Work out the finished part from the listing and answer in its coordinate system (mm). Face numbers are marked on the shaded views. A direction names the side the tool comes from. Coordinates: 2 decimals unless noted, no trailing zeros. Order: outer loops, then holes, each group sorted by start corner. A loop starts at its lowest first (then second) coordinate and runs counter-clockwise, first axis right, second up.
1. Determine the mould class of the marked faces 1, 2, 3 and 4 for opening direction X: +X half, -X half, draft (parallel to the pull), parting line (faces both ways), or undercut.
2. The part is cut by section B-B, the plane x = -6. Give the vertices of the cut face in (y, z), then the cut area to 3 significant figures.
3. Find the intervals of material crossed by probe 1 along X at (y, z) = (6, 0.45); probe 2 along Y at (x, z) = (-28.5, 2.15); probe 3 along Y at (x, z) = (-7.5, 2.1), in increasing order.
4. A tool of negligible diameter and unlimited length cuts with its end or side. For the marked faces 5, 6 and 7, from which of +Z, -Z, +X, -X, +Y, -Y can it reach the whole face along a straight path? Write none if from no direction.
5. The part is cut by section D-D, the plane y = 12. Give the vertices of the cut face in (x, z), then the cut area to 3 significant figures.
6. The part is cut by section C-C, the plane z = 2.15. Give the vertices of the cut face in (x, y), then the cut area to 3 significant figures.
7. The part is cut by section A-A, the plane y = 6. Give the vertices of the cut face in (x, z), then the cut area to 3 significant figures.
8. A flat-ended cylindrical pin translates along its axis: pin 1 Ø1.5 at (x, z) = (-9.5, 1) entering from +Y. Find the tip coordinate at first contact, or state that the pin passes through.
Autodesk Inventor part; units mm, degrees
ref_plane "YZ Plane" through (0, 0, 0) normal (1, 0, 0) x (0, 1, 0)
ref_plane "XZ Plane" through (0, 0, 0) normal (0, 1, 0) x (-1, 0, 0)
ref_plane "XY Plane" through (0, 0, 0) normal (0, 0, 1) x (1, 0, 0)
sketch "Sketch1" plane through (0, 0, 0) normal (0, 1, 0) x (-1, 0, 0)
  line L0 (0, 0) -> (34, 0)
  line L1 (34, 0) -> (34, 3)
  line L2 (34, 3) -> (0, 3)
  line L3 (0, 3) -> (0, 0)
  dimension "d0" = 34
  dimension "d1" = 3
extrude "Extrusion1" add sketch "Sketch1" along normal blind 10
sketch "Sketch2" plane through (0, 10, 0) normal (0, 1, 0) x (1, 0, 0)
  line L0 (-34, -3) -> (0, -3)
  line L1 (-34, 0) -> (-29, 0)
  line L2 (-29, 0) -> (-29, -3)
  line L3 (-29, -3) -> (-34, -3)
  line L4 (-34, -3) -> (-34, 0)
  line L5 (-5, 0) -> (0, 0)
  line L6 (0, 0) -> (0, -3)
  line L7 (0, -3) -> (-5, -3)
  line L8 (-5, -3) -> (-5, 0)
  line L9 (-19.5, 0) -> (-14.5, 0)
  line L10 (-14.5, 0) -> (-14.5, -3)
  line L11 (-14.5, -3) -> (-19.5, -3)
  line L12 (-19.5, -3) -> (-19.5, 0)
  dimension "d4" = 3
  dimension "d5" = 5
  dimension "d6" = 3
  dimension "d7" = 5
  dimension "d8" = 3
  dimension "d9" = 5
  dimension "d10" = 9.5
extrude "Extrusion2" add sketch "Sketch2" along normal blind 3
sketch "Sketch4" plane through (0, 0, 0) normal (0, 0, -1) x (-1, 0, 0)
  line L0 (34, 0) -> (34, 13)
  line L1 (30, 2.5) -> (27, 2.5)
  line L2 (27, 2.5) -> (27, 7.5)
  line L3 (27, 7.5) -> (30, 7.5)
  line L4 (30, 7.5) -> (30, 2.5)
  line L5 (0, 0) -> (34, 0)
  line L6 (0, 0) -> (0, 13)
  line L7 (17, 0) -> (17, 25.0309) construction
  line L8 (7, 2.5) -> (7, 7.5)
  line L9 (4, 2.5) -> (7, 2.5)
  line L10 (7, 7.5) -> (4, 7.5)
  line L11 (4, 7.5) -> (4, 2.5)
  line L12 (19.5, 10) -> (29, 10)
  dimension "d17" = 3
  dimension "d18" = 5
  dimension "d22" = 2.5
  dimension "d23" = 4
  dimension "d25" = 10
extrude "Extrusion4" cut sketch "Sketch4" against normal blind 3
equation "\"d22\" = -0.5 * d18 + 0.5 * d25"
properties part number "link2p1press" material "Glass"
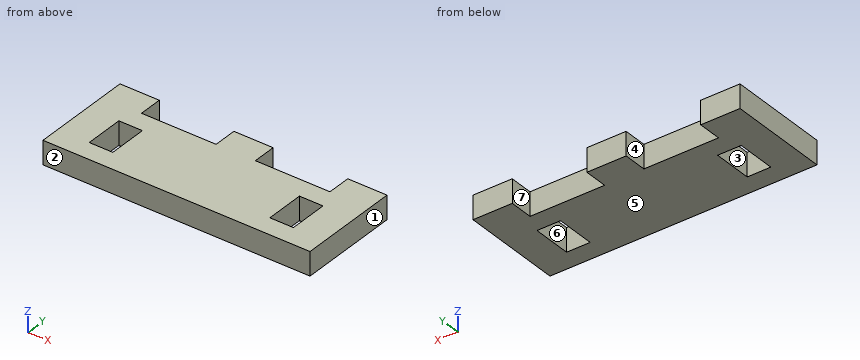
Geometry says:
1. face 1: +X half
1. face 2: draft
1. face 3: undercut
1. face 4: undercut
2. outline: (0, 0) - (2.5, 0) - (2.5, 3) - (0, 3) - close; (7.5, 0) - (10, 0) - (10, 3) - (7.5, 3) - close
2. area: 15.0 mm2
3. probe 1: x = -34 to -30, -27 to -7, -4 to 0
3. probe 2: y = 0 to 2.5, 7.5 to 10
3. probe 3: y = 0 to 10
4. face 5: -Z, +X, -X, +Y, -Y
4. face 6: +Z, -Z
4. face 7: +Z, -Z, +Y
5. outline: (-34, 0) - (-29, 0) - (-29, 3) - (-34, 3) - close; (-19.5, 0) - (-14.5, 0) - (-14.5, 3) - (-19.5, 3) - close; (-5, 0) - (0, 0) - (0, 3) - (-5, 3) - close
5. area: 45.0 mm2
6. outline: (-34, 0) - (0, 0) - (0, 13) - (-5, 13) - (-5, 10) - (-14.5, 10) - (-14.5, 13) - (-19.5, 13) - (-19.5, 10) - (-29, 10) - (-29, 13) - (-34, 13) - close; hole (-30, 2.5) - (-27, 2.5) - (-27, 7.5) - (-30, 7.5) - close; hole (-7, 2.5) - (-4, 2.5) - (-4, 7.5) - (-7, 7.5) - close
6. area: 355 mm2
7. outline: (-34, 0) - (-30, 0) - (-30, 3) - (-34, 3) - close; (-27, 0) - (-7, 0) - (-7, 3) - (-27, 3) - close; (-4, 0) - (0, 0) - (0, 3) - (-4, 3) - close
7. area: 84.0 mm2
8. pin 1: stops at y = 10
